Model file for the job. Use its own axes, mm. A direction names the side the tool comes from. Coordinates: 2 decimals unless noted, no trailing zeros. Order: outer loops, then holes, each group sorted by start corner. A loop starts at its lowest first (then second) coordinate and runs counter-clockwise, first axis right, second up.
from build123d import *

# Parameters (mm, degrees)
F1_DEPTH = 5.5
F2_DEPTH = 9.5
F3_W     = 12
F3_H     = 7
F4_DEPTH = 44.1
F6_DEPTH = 4
F8_DEPTH = 4
F9_R     = 5
F10_R    = 5
F11_R    = 5
F12_R    = 5


# Not quite as in the source:
# - a feature names something its author has since deleted; it is built from what else it names


with BuildPart() as f1:
    # F0 (on Top) → F1 (new body, symmetric)
    with BuildSketch(Plane.XY):
        Polygon((41.8999169252, -11.2350502836), (25.8999169252, -9.8352316672), (25.8999169252, -51.2350502836), (41.8999169252, -51.2350502836), align=None)
    extrude(amount=F1_DEPTH, both=True)

    # F0 (on Top) → F2 (join, symmetric)
    with BuildSketch(Plane.XY):
        Polygon((41.8999169252, -51.2350502836), (25.8999169252, -51.2350502836), (22.3999169252, -51.2350502836), (22.3999169252, -55.7350502836), (45.3999169252, -55.7350502836), (45.3999169252, -51.2350502836), align=None)
    extrude(amount=F2_DEPTH, both=True)

    # F3 (on face) → F4 (cut)
    with BuildSketch(Plane(origin=(0, -51.2350502836, 0), x_dir=(-1, 0, 0), z_dir=(0, 1, 0))):
        with Locations((-33.8999169252, 0)):
            Rectangle(F3_W, F3_H)
    extrude(amount=F4_DEPTH, mode=Mode.SUBTRACT)

    # F5 (on face) → F6 (join)
    with BuildSketch(Plane.XY.offset(5.5)):
        with BuildLine():
            Line((29.8999169252, -51.2350502836), (37.8999169252, -51.2350502836))
            ThreePointArc((37.8999169252, -51.2350502836), (33.8999169252, -47.2350502836), (29.8999169252, -51.2350502836))
        make_face()
    extrude(amount=F6_DEPTH)

    # F7 (on face) → F8 (join)
    with BuildSketch(Plane(origin=(0, 0, -5.5), x_dir=(1, 0, 0), z_dir=(0, 0, -1))):
        with BuildLine():
            ThreePointArc((29.8999169252, 51.2350502836), (33.8999169252, 47.2350502836), (37.8999169252, 51.2350502836))
            Line((37.8999169252, 51.2350502836), (29.8999169252, 51.2350502836))
        make_face()
    extrude(amount=F8_DEPTH)

    # F9
    f9_edges = [f1.edges().sort_by_distance(p)[0] for p in [
        (22.399917, -53.48505, 9.5),
    ]]
    fillet(f9_edges, radius=F9_R)

    # F10
    f10_edges = [f1.edges().sort_by_distance(p)[0] for p in [
        (45.399917, -53.48505, 9.5),
    ]]
    fillet(f10_edges, radius=F10_R)

    # F11
    f11_edges = [f1.edges().sort_by_distance(p)[0] for p in [
        (45.399917, -53.48505, -9.5),
    ]]
    fillet(f11_edges, radius=F11_R)

    # F12
    f12_edges = [f1.edges().sort_by_distance(p)[0] for p in [
        (22.399917, -53.48505, -9.5),
    ]]
    fillet(f12_edges, radius=F12_R)


solid = f1.part
Q1. Cut at C-C, the plane y = -52.5. List the corners of the cut face in (x, z).
Established:
outline: (22.4, -4.5) arc R5 ccw to (27.4, -9.5) - (40.4, -9.5) arc R5 ccw to (45.4, -4.5) - (45.4, 4.5) arc R5 ccw to (40.4, 9.5) - (27.4, 9.5) arc R5 ccw to (22.4, 4.5) - close
Q2. Cut at A-A, the plane y = -35. List the corners of the cut face in (x, z), plus the area to 3 significant figures.
Established:
outline: (25.9, -5.5) - (41.9, -5.5) - (41.9, 5.5) - (25.9, 5.5) - close; hole (27.9, -3.5) - (39.9, -3.5) - (39.9, 3.5) - (27.9, 3.5) - close
area: 92.0 mm2
Q3. Cut at B-B, the plane z = -2. List the corners of the cut face in (x, y).
Established:
outline: (22.4, -55.74) - (45.4, -55.74) - (45.4, -51.24) - (41.9, -51.24) - (41.9, -11.24) - (39.9, -11.06) - (39.9, -51.24) - (27.9, -51.24) - (27.9, -10.01) - (25.9, -9.84) - (25.9, -51.24) - (22.4, -51.24) - close
Q4. Probe line 1 (Z direction, x = 38, y = -34); line 2 (X direction, y = -39.5, z = -3); line 3 (X direction, y = -41, z = 4.75). List the from-to ranges inside material, lowest first.
Established:
line 1: z = -5.5 to -3.5, 3.5 to 5.5
line 2: x = 25.9 to 27.9, 39.9 to 41.9
line 3: x = 25.9 to 41.9
Q5. Cut at D-D, the plane x = 38.5. List the corners of the cut face in (y, z).
Established:
outline: (-55.74, -9.5) - (-51.24, -9.5) - (-51.24, -5.5) - (-10.94, -5.5) - (-10.94, -3.5) - (-51.24, -3.5) - (-51.24, 3.5) - (-10.94, 3.5) - (-10.94, 5.5) - (-51.24, 5.5) - (-51.24, 9.5) - (-55.74, 9.5) - close
Q6. Which spindle directions (+Z, -Z, +X, -X, +Y, -Y) get a long thin tool onto all of the face, cutting with end or side? Do faces 1 (the face through (25.9, -30, 0)), 2 (the face through (33.988, -47.236, 7.472)), 3 (the face through (41.9, -32, 0)), 4 (the face through (34, -31, -3.5)). Say none if no direction does.
Established:
face 1: +Z, -Z, -X, +Y
face 2: +Z, +Y
face 3: +Z, -Z, +X, +Y
face 4: +Y
Q7. Drop flat-ended pins along their axis: P1, Ø3.5, axis at x = 36.5, y = -36.5, coming from the -Z side; P2, Ø6, axis at x = 39.5, y = -23.5, coming from the +Z side; P3, Ø7.5, axis at y = -34, z = 1.5, coming from the +X side. Give the stop position or say it passes through.
Established:
P1: stops at z = -5.5
P2: stops at z = 5.5
P3: stops at x = 41.9
Q8. Mould opens along X. For faces 5 (the face through (34, -31, 3.5)), 6 (the face through (39.9, -31, 0)), 7 (the face through (25, -51.235, 0)), 8 (the face through (23.9, -53.52, -8.07)) say: pulls with the +X half, pulls with the -X half, needs draft (parallel to the pull), parting line crosses it, or undercut.
Established:
face 5: undercut
face 6: undercut
face 7: needs draft
face 8: pulls with the -X half
